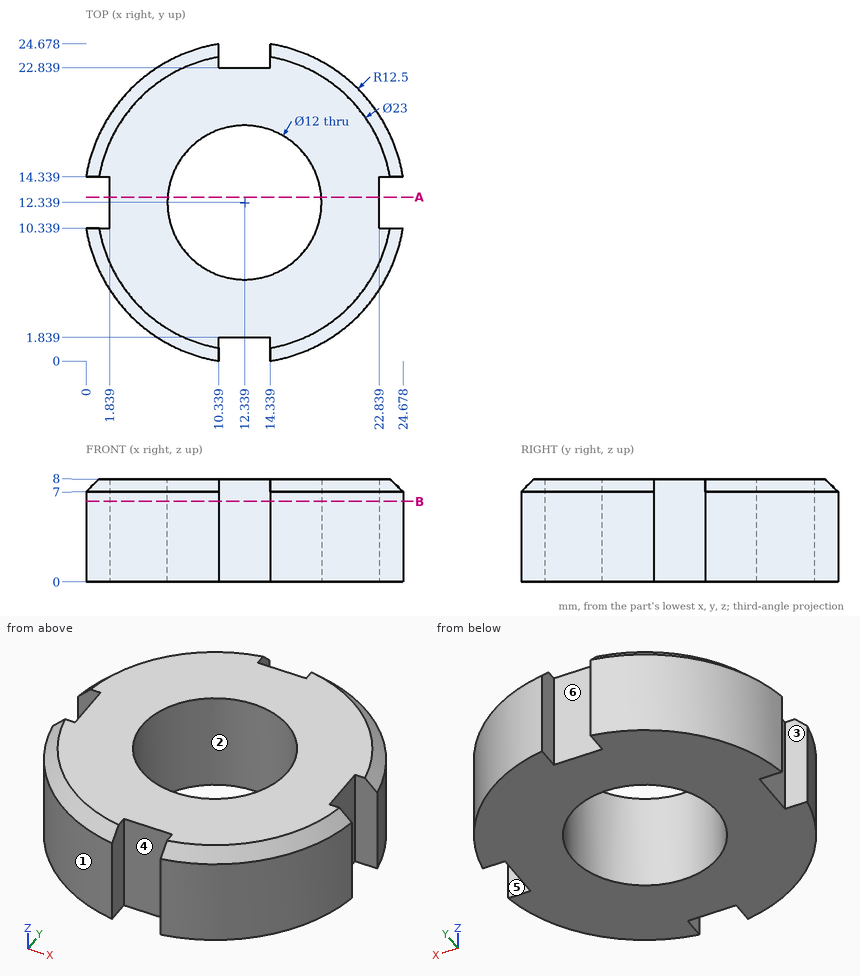
Print and shaded views of the part. All mm, measured from the part's lowest x, y and z. A direction names the side the tool comes from. Coordinates: 2 decimals unless noted, no trailing zeros. Order: outer loops, then holes, each group sorted by start corner. A loop starts at its lowest first (then second) coordinate and runs counter-clockwise, first axis right, second up. Notation, with made-up numbers: (-14.75, 17) -> (-1.75, 17) arc R10 ccw to (-1.75, 25) -> close; hole circle Ø9 at (85, -8). An arc over 180 degrees is marked (long way). Answer as a JSON object with one key per item and string values. Group by question number.
1) Cut at B-B, the plane z = 6.25. Write the cut outline in (x, y), then the cut area to 3 significant figures.
2) Pull direction X, two halves, no side cores. Call the marked faces 1, 2 and 3: +X half, -X half, draft (parallel to the pull), parting line (faces both ways), or undercut.
3) Flat gauge pins, fed straight in: pin 1 (5 mm diameter, centred on x = 17, y = 9, fed in from -Z); pin 2 (2 mm diameter, centred on x = 24, z = 2, fed in from +Y) (1 decimal); pin 3 (1.2 mm diameter, centred on y = 13, z = 5.5, fed in from -X); pin 4 (3 mm diameter, centred on x = 12, z = 4, fed in from +Y). Where does each tip first touch, or does it go through?
4) Which spindle directions (+Z, -Z, +X, -X, +Y, -Y) get a long thin tool onto all of the face, cutting with end or side? Do the marked faces 4, 5 and 6. Say none if no direction does.
5) Cut at A-A, the plane y = 12.75. Write the cut outline in (x, z) (3 decimals), then the cut area to 3 significant figures.
6) Drill centre lines: L1, parallel to Y at x = 12.5, z = 2.25; L2, parallel to X at y = 11.25, z = 3.75; L3, parallel to Y at x = 16.75, z = 5.5 (1 decimal). Where is each one in solid material? Low to high.
Check values:
{
 "1": {"outline": "(0, 10.34) arc R12.5 ccw to (10.34, 0) -> (10.34, 1.84) -> (14.34, 1.84) -> (14.34, 0) arc R12.5 ccw to (24.68, 10.34) -> (22.84, 10.34) -> (22.84, 14.34) -> (24.68, 14.34) arc R12.5 ccw to (14.34, 24.68) -> (14.34, 22.84) -> (10.34, 22.84) -> (10.34, 24.68) arc R12.5 ccw to (0, 14.34) -> (1.84, 14.34) -> (1.84, 10.34) -> close; hole circle Ø12 at (12.34, 12.34)", "area": "347 mm²"},
 "2": {"face 1": "-X half", "face 2": "undercut", "face 3": "draft"},
 "3": {"pin 1": "stops at z = 0", "pin 2": "stops at y = 18.9", "pin 3": "stops at x = 1.84", "pin 4": "stops at y = 22.84"},
 "4": {"face 4": "+Z, -Z, -Y", "face 5": "+Z, -Z, +X", "face 6": "+Z, -Z, +Y"},
 "5": {"outline": "(1.839, 0) -> (6.353, 0) -> (6.353, 8) -> (1.839, 8) -> close; (18.325, 0) -> (22.839, 0) -> (22.839, 8) -> (18.325, 8) -> close", "area": "72.2 mm²"},
 "6": {"L1": "y = 1.84 to 6.34, 18.34 to 22.84", "L2": "x = 1.84 to 6.44, 18.24 to 22.84", "L3": "y = 0.6 to 8.3, 16.4 to 24"}
}
